Work out the finished part from the listing and answer in its coordinate system (mm). A direction names the side the tool comes from. Give positions to 0.01 mm unless a question says otherwise; leave off trailing zeros. Loops run counter-clockwise (first coordinate to the right, second up) from the corner with the lowest first, then second, coordinate; pieces in that order, holes last. Notation, with made-up numbers: M -25.75,30 L 18.25,30 A15 cw 18.25,48 Z; hole C 44.25,-23.75 d2. An arc over 180 degrees is marked long. Answer as a JSON object with one key per item and string values. Group by question number.
```python
from build123d import *

# Parameters (mm, degrees)
SKETCH_1_R                = 38
SKETCH_1_R_2              = 14
EXTRUDE_1_DEPTH           = 10
HOLE_WIZARD_1_D           = 3.2
HOLE_WIZARD_1_CBORE_D     = 6
HOLE_WIZARD_1_CBORE_DEPTH = 3.4
HOLE_WIZARD_4_0_4_1_D     = 4
CHAMFER_1_SIZE            = 1


with BuildPart() as part:
    # 草图1 → 凸台-拉伸1 (new body)
    with BuildSketch(Plane.XY):
        Circle(SKETCH_1_R)
        Circle(SKETCH_1_R_2, mode=Mode.SUBTRACT)
    extrude(amount=EXTRUDE_1_DEPTH)

    # 打孔尺寸(%根据)内六角圆柱头螺钉的类型1 (through all)
    with Locations(Plane.XY.offset(10)):
        with Locations((0, 34.5), (34.5, 0), (0, -34.5), (-34.5, 0)):
            CounterBoreHole(HOLE_WIZARD_1_D / 2, HOLE_WIZARD_1_CBORE_D / 2, HOLE_WIZARD_1_CBORE_DEPTH)

    # Ø4.0 (4) 直径孔1 (through all)
    with Locations(Plane(origin=(0, 0, 0), x_dir=(-1, 0, 0), z_dir=(0, 0, -1))):
        with Locations((29, 0)):
            Hole(HOLE_WIZARD_4_0_4_1_D / 2)

    # 倒角1
    # the kernel refuses this chamfer: 1 mm, written as the material it takes off along each edge
    with BuildSketch(Plane(origin=(-29, 0, 0), x_dir=(1, 0, 0), z_dir=(0, -1, 0))) as chamfer_1_piece_1:
        Polygon((2 + CHAMFER_1_SIZE, 0), (2, CHAMFER_1_SIZE), (2, 0), align=None)
    revolve(axis=Axis((-29, 0, 0), (0, 0, 1)), mode=Mode.SUBTRACT)
    with BuildSketch(Plane(origin=(-29, 0, 10), x_dir=(1, 0, 0), z_dir=(0, -1, 0))) as chamfer_1_piece_2:
        Polygon((2 + CHAMFER_1_SIZE, 0), (2, -CHAMFER_1_SIZE), (2, 0), align=None)
    revolve(axis=Axis((-29, 0, 10), (0, 0, 1)), mode=Mode.SUBTRACT)


solid = part.part
```
Item 1: A cutting plane is placed at D-D (x = -34.5). Determine the outline of the cut face in (y, z).
Item 2: A cutting plane is placed at C-C (z = 4.5). Determine the outline of the cut face in (x, y), and give its area (3 significant figures).
Item 3: A cutting plane is placed at B-B (x = 0). Determine the outline of the cut face in (y, z).
Item 4: A tool of negligible diameter and unlimited length cuts with its end or side. For faces 1 (the cylindrical face through (12.932, -5.362, 4.93)), 2 (the cylindrical face through (-37.5, 0.1, 8.3)), from which of +Z, -Z, +X, -X, +Y, -Y can it reach the whole face along a straight path? Write none if from no direction.
Item 5: For a pull along Y with two mould halves and no side action, classify faces 3 (the cylindrical face through (31.5, 0.1, 8.3)), 4 (the flat face through (16, 1, 0)), 5 (the cylindrical face through (17.535, -33.713, 4.93)) as pulls with the +Y half, pulls with the -Y half, needs draft (parallel to the pull), parting line crosses it, or undercut.
Item 6: Find the intervals of material crossed by probe 1 along Y at (x, z) = (0, 7.8); probe 2 along Y at (x, z) = (34.5, 2); probe 3 along Y at (x, z) = (-8, 8.5), in increasing order. Write a range as [from, to].
Item 7: Given pin 1 Ø1.8 at (x, y) = (34.5, 1) entering from +Z; pin 2 Ø3 at (x, y) = (0, 34.5) entering from -Z; pin 3 Ø5 at (y, z) = (-15, 5) entering from -X; pin 4 Ø1.5 at (x, z) = (12.5, 4.5) entering from -Y, each flat-ended and moving along its own axis, determine where each tip first touches the part or whether it passes through.
Item 8: A cutting plane is placed at A-A (y = 0). Give the number of separate pieces and of enclosed holes in the cut face, and give its area (3 significant figures).
The answers:
{
 "1": {"outline": "M -15.93,0 L -1.6,0 L -1.6,6.6 L -3,6.6 L -3,10 L -15.93,10 Z; M 1.6,0 L 15.93,0 L 15.93,10 L 3,10 L 3,6.6 L 1.6,6.6 Z"},
 "2": {"outline": "C 0,0 d76; hole C -34.5,0 d3.2; hole C -29,0 d4; hole C 0,0 d28; hole C 0,-34.5 d3.2; hole C 0,34.5 d3.2; hole C 34.5,0 d3.2", "area": "3,880 mm^2"},
 "3": {"outline": "M -38,0 L -36.1,0 L -36.1,6.6 L -37.5,6.6 L -37.5,10 L -38,10 Z; M -32.9,0 L -14,0 L -14,10 L -31.5,10 L -31.5,6.6 L -32.9,6.6 Z; M 14,0 L 32.9,0 L 32.9,6.6 L 31.5,6.6 L 31.5,10 L 14,10 Z; M 36.1,0 L 38,0 L 38,10 L 37.5,10 L 37.5,6.6 L 36.1,6.6 Z"},
 "4": {"face 1": "+Z, -Z", "face 2": "+Z"},
 "5": {"face 3": "undercut", "face 4": "needs draft", "face 5": "parting line crosses it"},
 "6": {"probe 1": "y = [-38, -37.5], [-31.5, -14], [14, 31.5], [37.5, 38]", "probe 2": "y = [-15.93, -1.6], [1.6, 15.93]", "probe 3": "y = [-37.15, -11.49], [11.49, 37.15]"},
 "7": {"pin 1": "stops at z = 6.6", "pin 2": "passes through", "pin 3": "stops at x = -35.89", "pin 4": "stops at y = -36.14"},
 "8": {"separate pieces": "5", "enclosed holes": "0", "area": "355 mm^2"}
}
